from build123d import *

# Parameters (mm, degrees)
F0_W     = 76.2
F0_H     = 76.2
F1_DEPTH = 609.6
F3_DEPTH = 914.4
F4_DEPTH = 304.8
F5_DEPTH = 584.2


with BuildPart() as f1:
    # F0 (on Front) → F1 (new body)
    with BuildSketch(Plane.XZ):
        with Locations((-79.1539917648, 51.4746750653)):
            Rectangle(F0_W, F0_H)
    extrude(amount=F1_DEPTH)

    # F2 (on face) → F3 (cut)
    with BuildSketch(Plane.XZ.offset(609.6)):
        Polygon((-42.3204526305, 88.3055701852), (-98.6881405115, 88.3055701852), (-115.9909814596, 88.3055701852), (-115.9909814596, 14.655277133), (-42.3204526305, 14.655277133), align=None)
    extrude(amount=-F3_DEPTH, mode=Mode.SUBTRACT)

    # F4 (add): a face of the model
    f4_faces = [f1.faces().sort_by_distance(p)[0] for p in [
        (-42.1316224993, -609.6, 51.4746750653),
    ]]
    extrude(f4_faces, amount=F4_DEPTH)

    # F5 (add): a face of the model
    f5_faces = [f1.faces().sort_by_distance(p)[0] for p in [
        (-42.1316224993, 0, 51.4746750653),
    ]]
    extrude(f5_faces, amount=F5_DEPTH)


solid = f1.part
Source: CAD feature listing. Evaluate the final solid. Frame: model axes, mm. A direction names the side the tool comes from. Coordinates: 2 decimals unless noted, no trailing zeros. Loops run counter-clockwise (first coordinate to the right, second up) from the corner with the lowest first, then second, coordinate; pieces in that order, holes last. Notation, with made-up numbers: (40.5, -37.5) - (79.5, -37.5) arc R16 cw to (79.5, -7.5) - close; hole circle Ø6 at (-24.5, -32). An arc over 180 degrees is marked (long way). One line per item, written item: value. Start each with the question number.
1. Section B-B (x = -58). Return the cut outline in (y, z).
2. Set-up query: faces 1 (the flat face through (-42.32, -176, 51)), 2 (the flat face through (-117.254, -176, 51)). Return all of +Z, -Z, +X, -X, +Y, -Y with unobstructed straight access to the full face (end or side cutting, diameter ignored); none if empty.
3. Mould query, pull axis X, two halves, no side actions, for faces 3 (the flat face through (-80, -176, 13.375)), 4 (the flat face through (-41.054, -176, 51)), 5 (the flat face through (-115.991, -176, 52)). Classes: pulls with the +X half, pulls with the -X half, needs draft (parallel to the pull), parting line crosses it, or undercut.
4. Ray query, L1, parallel to Z at x = -55.5, y = -224; L2, parallel to X at y = -50.5, z = 83.5. Return the intervals inside material, ascending.
5. Section C-C (y = -615). Return the cut outline in (x, z).
6. Section A-A (z = 64.5). Return the cut outline in (x, y), and give its area (3 significant figures).
Verdict:
1. outline: (-914.4, 13.37) - (584.2, 13.37) - (584.2, 14.66) - (-914.4, 14.66) - close; (-914.4, 88.31) - (584.2, 88.31) - (584.2, 89.57) - (-914.4, 89.57) - close
2. face 1: +Y, -Y
2. face 2: +Z, -Z, -X, +Y, -Y
3. face 3: needs draft
3. face 4: pulls with the +X half
3. face 5: undercut
4. L1: z = 13.37 to 14.66, 88.31 to 89.57
4. L2: x = -117.25 to -115.99, -42.32 to -41.05
5. outline: (-117.25, 13.37) - (-41.05, 13.37) - (-41.05, 89.57) - (-117.25, 89.57) - close; hole (-115.99, 14.66) - (-42.32, 14.66) - (-42.32, 88.31) - (-115.99, 88.31) - close
6. outline: (-117.25, -914.4) - (-115.99, -914.4) - (-115.99, 584.2) - (-117.25, 584.2) - close; (-42.32, -914.4) - (-41.05, -914.4) - (-41.05, 584.2) - (-42.32, 584.2) - close
6. area: 3,790 mm2
